from build123d import *

# Parameters (mm, degrees)
ESQUISSE1_W             = 198
ESQUISSE1_H             = 320
BOSS_EXTRU_1_DEPTH      = 3
ENL_V_MAT_EXTRU_1_REACH = 194.445
ESQUISSE2_R             = 2.2
ENL_V_MAT_EXTRU_3_REACH = 194.445


with BuildPart() as part:
    # Esquisse1 → Boss.-Extru.1 (new body)
    with BuildSketch(Plane.XY):
        with Locations((0, 5)):
            Rectangle(ESQUISSE1_W, ESQUISSE1_H)
    extrude(amount=BOSS_EXTRU_1_DEPTH)

    # Esquisse2 → Enlèv. mat.-Extru.1 (cut, up to next)
    with BuildSketch(Plane.XY.offset(3), mode=Mode.PRIVATE) as enl_v_mat_extru_1_sk1:
        with Locations((9, -145)):
            Circle(ESQUISSE2_R)
    enl_v_mat_extru_1_tool1 = extrude(enl_v_mat_extru_1_sk1.sketch, amount=-ENL_V_MAT_EXTRU_1_REACH, mode=Mode.PRIVATE) & part.part
    # Esquisse2 → Enlèv. mat.-Extru.1 (cut, up to next)
    with BuildSketch(Plane.XY.offset(3), mode=Mode.PRIVATE) as enl_v_mat_extru_1_sk2:
        with Locations((-9, -145)):
            Circle(ESQUISSE2_R)
    enl_v_mat_extru_1_tool2 = extrude(enl_v_mat_extru_1_sk2.sketch, amount=-ENL_V_MAT_EXTRU_1_REACH, mode=Mode.PRIVATE) & part.part
    # Esquisse2 → Enlèv. mat.-Extru.1 (cut, up to next)
    with BuildSketch(Plane.XY.offset(3), mode=Mode.PRIVATE) as enl_v_mat_extru_1_sk3:
        with Locations((-9, 155)):
            Circle(ESQUISSE2_R)
    enl_v_mat_extru_1_tool3 = extrude(enl_v_mat_extru_1_sk3.sketch, amount=-ENL_V_MAT_EXTRU_1_REACH, mode=Mode.PRIVATE) & part.part
    # Esquisse2 → Enlèv. mat.-Extru.1 (cut, up to next)
    with BuildSketch(Plane.XY.offset(3), mode=Mode.PRIVATE) as enl_v_mat_extru_1_sk4:
        with Locations((9, 155)):
            Circle(ESQUISSE2_R)
    enl_v_mat_extru_1_tool4 = extrude(enl_v_mat_extru_1_sk4.sketch, amount=-ENL_V_MAT_EXTRU_1_REACH, mode=Mode.PRIVATE) & part.part
    add(enl_v_mat_extru_1_tool1.solids().sort_by_distance((9, -145, 3))[0], mode=Mode.SUBTRACT)
    add(enl_v_mat_extru_1_tool2.solids().sort_by_distance((-9, -145, 3))[0], mode=Mode.SUBTRACT)
    add(enl_v_mat_extru_1_tool3.solids().sort_by_distance((-9, 155, 3))[0], mode=Mode.SUBTRACT)
    add(enl_v_mat_extru_1_tool4.solids().sort_by_distance((9, 155, 3))[0], mode=Mode.SUBTRACT)

    # Esquisse5 → Enlèv. mat.-Extru.3 (cut, up to next)
    with BuildSketch(Plane.XY.offset(3), mode=Mode.PRIVATE) as enl_v_mat_extru_3_sk1:
        Polygon((0, 22), (26, 22), (26, 55), (16, 65), (-17, 65), (-26, 56), (-26, 22), align=None)
    enl_v_mat_extru_3_tool1 = extrude(enl_v_mat_extru_3_sk1.sketch, amount=-ENL_V_MAT_EXTRU_3_REACH, mode=Mode.PRIVATE) & part.part
    add(enl_v_mat_extru_3_tool1.solids().sort_by_distance((-0.094073, 42.727414, 3))[0], mode=Mode.SUBTRACT)


solid = part.part
Could you check a few things on this model? Use its own coordinates, in mm. A direction names the side the tool comes from. Coordinates: 2 decimals unless noted, no trailing zeros. Order: outer loops, then holes, each group sorted by start corner. A loop starts at its lowest first (then second) coordinate and runs counter-clockwise, first axis right, second up.
Q1. Thinking about a two-plate mould opening in Y: for faces 3 (the flat face through (-1, 7, 3)), 4 (the flat face through (-21, 61, 2)), which applies, released by +Y, released by -Y, zero draft, split by the parting line, or undercut?
Q2. Suppose I cut it at B-B on z = 1.5. Please give me the cut outline in (x, y).
Q3. Which directions (+Z, -Z, +X, -X, +Y, -Y) give clear straight access to the entire face, cutting with the end or side of a thin tool? Please do faces 1 (the flat face through (-1, 7, 0)), 2 (the flat face through (21, 60, 2)).
Q4. Will this pin go through, and if not, where does the flat tip stop? pin 1 (2.5 mm diameter, centred on x = -9, y = -145, fed in from -Z).
Q5. Please list where these lines run through material, in increasing order: L1, parallel to Y at x = -9, z = 0.75; L2, parallel to X at y = -145, z = 2.15; L3, parallel to Y at x = 11, z = 0.65.
Q6. Suppose I cut it at A-A on y = 61.5. Please give me the cut outline in (x, z).
Answer:
1. face 3: zero draft
1. face 4: undercut
2. outline: (-99, -155) - (99, -155) - (99, 165) - (-99, 165) - close; hole (-26, 22) - (26, 22) - (26, 55) - (16, 65) - (-17, 65) - (-26, 56) - close; hole circle Ø4.4 at (-9, -145); hole circle Ø4.4 at (-9, 155); hole circle Ø4.4 at (9, -145); hole circle Ø4.4 at (9, 155)
3. face 1: -Z, +X, -X, +Y, -Y
3. face 2: +Z, -Z
4. pin 1: passes through
5. L1: y = -155 to -147.2, -142.8 to 22, 65 to 152.8, 157.2 to 165
5. L2: x = -99 to -11.2, -6.8 to 6.8, 11.2 to 99
5. L3: y = -155 to -145.92, -144.08 to 22, 65 to 154.08, 155.92 to 165
6. outline: (-99, 0) - (-20.5, 0) - (-20.5, 3) - (-99, 3) - close; (19.5, 0) - (99, 0) - (99, 3) - (19.5, 3) - close
